```python
from build123d import *

# Parameters (mm, degrees)
BOSS_EXTRUDE1_DEPTH = 10
CUT_EXTRUDE1_START  = -10
SKETCH2_R           = 1.5
CUT_EXTRUDE1_DEPTH  = 0.8
CUT_EXTRUDE2_START  = -15
SKETCH2_3_R         = 1.5
CUT_EXTRUDE2_DEPTH  = 15
CUT_EXTRUDE3_DEPTH  = 76.909294374


with BuildPart() as part:
    # Sketch1 → Boss-Extrude1 (new body)
    # profile 1 of 2: a face of its own
    with BuildSketch(Plane(origin=(0, 0, 0), x_dir=(1, 0, 0), z_dir=(0, 1, 0))):
        Polygon((71.317746546, -5), (48.423009704, 24), (12.576990296, 24), (-10.317746546, -5), align=None)
        Polygon((15, 19), (0, 0), (61, 0), (46, 19), align=None, mode=Mode.SUBTRACT)
    # profile 2 of 2: a face of its own
    with BuildSketch(Plane(origin=(0, 0, 0), x_dir=(1, 0, 0), z_dir=(0, 1, 0))):
        Polygon((46, 19), (15, 19), (0, 0), (61, 0), align=None)
    extrude(amount=BOSS_EXTRUDE1_DEPTH)

    # Sketch2 → Cut-Extrude1 (cut)
    with BuildSketch(Plane.XZ.offset(CUT_EXTRUDE1_START)):
        Polygon((14.75769903, -19.5), (46.24230097, -19.5), (62.031774655, 0.5), (-1.031774655, 0.5), align=None)
        with Locations(Location((27.35, -16.5, 0), (0, 0, 90))):
            Circle(SKETCH2_R, mode=Mode.SUBTRACT)
        with Locations(Location((33.65, -16.5, 0), (0, 0, 90))):
            Circle(SKETCH2_R, mode=Mode.SUBTRACT)
    extrude(amount=CUT_EXTRUDE1_DEPTH, mode=Mode.SUBTRACT)

    # Sketch2<3> → Cut-Extrude2 (cut)
    with BuildSketch(Plane.XZ.offset(CUT_EXTRUDE2_START)):
        with Locations(Location((27.35, -16.5, 0), (0, 0, 270))):
            Circle(SKETCH2_3_R)
        with Locations(Location((33.65, -16.5, 0), (0, 0, 270))):
            Circle(SKETCH2_3_R)
    extrude(amount=CUT_EXTRUDE2_DEPTH, mode=Mode.SUBTRACT)

    # Sketch3 → Cut-Extrude3 (cut, through all)
    with BuildSketch(Plane.XZ):
        Polygon((40.330212267, 5), (40.330212267, -24), (48.423009704, -24), (71.317746546, 5), align=None)
    extrude(amount=-CUT_EXTRUDE3_DEPTH, mode=Mode.SUBTRACT)


solid = part.part
```
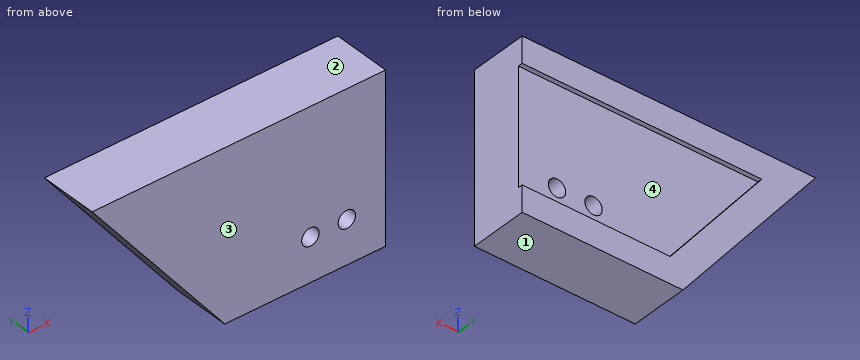
Here's how the part is built. I have some questions about the finished solid (model axes, mm). Face numbers are marked on the shaded views. Give positions to 0.01 mm unless a question says otherwise; leave off trailing zeros. Order: outer loops, then holes, each group sorted by start corner. A loop starts at its lowest first (then second) coordinate and runs counter-clockwise, first axis right, second up. Notation, with made-up numbers: (41, -30.75) - (92, -30.75) arc R14 cw to (92, -24.75) - close; hole circle Ø7 at (-12.75, 48). An arc over 180 degrees is marked (long way). Answer as a JSON object with one key per item and string values. Group by question number.
Item 1: If we section it at D-D on x = 1.5: Please give me the cut outline in (y, z), and give its area (3 significant figures).
Item 2: If we section it at A-A on x = 27.35: Please give me the cut outline in (y, z), and give its area (3 significant figures).
Item 3: If we section it at B-B on y = 7.25: Please give me the cut outline in (x, z), and give its area (3 significant figures).
Item 4: For P1, Ø2, axis at x = 2.5, y = 4, coming from the -Z side; P2, Ø6, axis at x = 14, z = -10, coming from the +Y side; P3, Ø1, axis at x = 5, y = 5, coming from the -Z side, each with a flat end and sliding along its axis, tell me the tip position at first contact or that it passes through.
Item 5: If we mould it in two halves opening along Z, with no side actions, what happens to the marked faces 1, 2, 3 and 4? For each: pulls with the +Z half, pulls with the -Z half, needs draft (parallel to the pull), parting line crosses it, or undercut.
Item 6: If we section it at C-C on z = -16.5: Please give me the cut outline in (x, y), and give its area (3 significant figures).
Item 7: Please list where these lines run through material, in increasing order: probe 1 along Z at (x, y) = (33.65, 5.5); probe 2 along X at (y, z) = (7.25, -16.5); probe 3 along Z at (x, y) = (19, 9.75).
Result set:
{
 "1": {"outline": "(0, -9.97) - (10, -9.97) - (10, -2.71) - (9.2, -2.71) - (9.2, 0.5) - (10, 0.5) - (10, 5) - (0, 5) - close", "area": "147 mm²"},
 "2": {"outline": "(0, -24) - (10, -24) - (10, -19.5) - (9.2, -19.5) - (9.2, -18) - (0, -18) - close; (0, -15) - (9.2, -15) - (9.2, 0.5) - (10, 0.5) - (10, 5) - (0, 5) - close", "area": "246 mm²"},
 "3": {"outline": "(-10.32, 5) - (12.58, -24) - (40.33, -24) - (40.33, 5) - close; hole circle Ø3 at (27.35, -16.5); hole circle Ø3 at (33.65, -16.5)", "area": "1,120 mm²"},
 "4": {"P1": "z = -12.5", "P2": "y = 9.2", "P3": "z = -15.04"},
 "5": {"face 1": "pulls with the -Z half", "face 2": "pulls with the +Z half", "face 3": "needs draft", "face 4": "undercut"},
 "6": {"outline": "(6.66, 0) - (25.85, 0) - (25.85, 9.2) - (12.39, 9.2) - (12.39, 10) - (6.66, 10) - close; (28.85, 0) - (32.15, 0) - (32.15, 9.2) - (28.85, 9.2) - close; (35.15, 0) - (40.33, 0) - (40.33, 9.2) - (35.15, 9.2) - close", "area": "259 mm²"},
 "7": {"probe 1": "-24 to -18, -15 to 5", "probe 2": "6.66 to 25.85, 28.85 to 32.15, 35.15 to 40.33", "probe 3": "-24 to -19.5, 0.5 to 5"}
}
